Check sheet for the drawn part. Datum: minimum x, y, z corner. Units: mm. A direction names the side the tool comes from. Give positions to 0.01 mm unless a question says otherwise; leave off trailing zeros. Order: outer loops, then holes, each group sorted by start corner. A loop starts at its lowest first (then second) coordinate and runs counter-clockwise, first axis right, second up. Notation, with made-up numbers: (64.25, -2) -> (84.25, -2) arc R31 cw to (84.25, 23) -> close; hole circle Ø8 at (85.5, 23.25). An arc over 180 degrees is marked (long way). One line per question, with ' | ' between items. Start each with the question number.
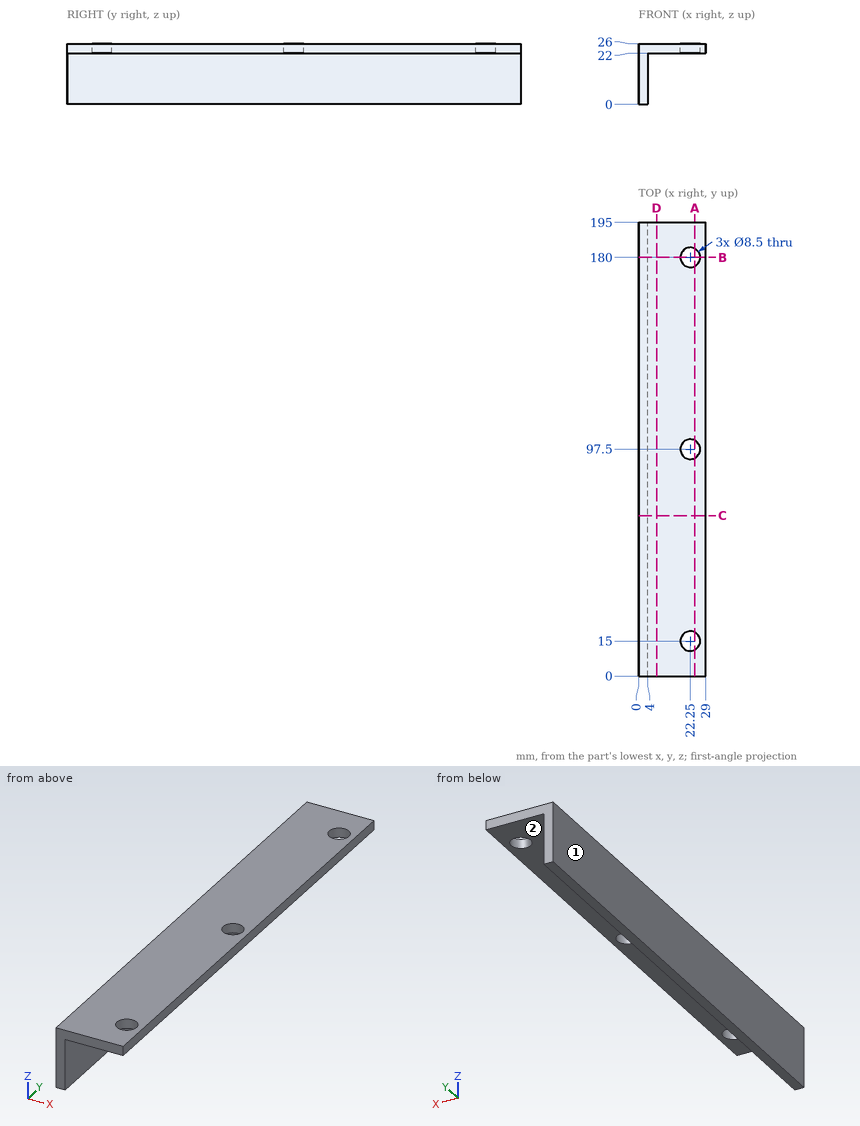
1. Cross-section at C-C on y = 69. Record the boundary of the cut face in (x, z).
2. Tool access check on the marked faces 1 and 2. Record the directions out of +Z, -Z, +X, -X, +Y, -Y that give a thin tool (end or side, any length) a straight path to the whole face; none if there is none.
3. Cross-section at D-D on x = 7.75. Record the boundary of the cut face in (y, z).
4. Cross-section at B-B on y = 180. Record the boundary of the cut face in (x, z), and give its area (3 significant figures).
5. Go/stop test with flat-tipped pins: pin 1 (13.5 mm diameter, centred on x = 22.25, y = 97.5, fed in from -Z); pin 2 (5 mm diameter, centred on y = 101, z = 10, fed in from +X). Record where each tip stops, or that it passes through.
6. Cross-section at A-A on x = 24.25. Record the boundary of the cut face in (y, z).
7. Scan lines: probe 1 along Y at (x, z) = (22.25, 23.2); probe 2 along Z at (x, y) = (21.25, 9.5); probe 3 along X at (y, z) = (35, 6.25). Record each from-to range of solid material in increasing order.
Response values:
1) outline: (0, 0) -> (4, 0) -> (4, 22) -> (29, 22) -> (29, 26) -> (0, 26) -> close
2) face 1: +Z, -Z, -X, +Y, -Y | face 2: -Z, +X, +Y, -Y
3) outline: (0, 22) -> (195, 22) -> (195, 26) -> (0, 26) -> close
4) outline: (0, 0) -> (4, 0) -> (4, 22) -> (18, 22) -> (18, 26) -> (0, 26) -> close; (26.5, 22) -> (29, 22) -> (29, 26) -> (26.5, 26) -> close | area: 170 mm²
5) pin 1: stops at z = 22 | pin 2: stops at x = 4
6) outline: (0, 22) -> (11.25, 22) -> (11.25, 26) -> (0, 26) -> close; (18.75, 22) -> (93.75, 22) -> (93.75, 26) -> (18.75, 26) -> close; (101.25, 22) -> (176.25, 22) -> (176.25, 26) -> (101.25, 26) -> close; (183.75, 22) -> (195, 22) -> (195, 26) -> (183.75, 26) -> close
7) probe 1: y = 0 to 10.75, 19.25 to 93.25, 101.75 to 175.75, 184.25 to 195 | probe 2: z = 22 to 26 | probe 3: x = 0 to 4
